Can you work these out from the model? Positions are in its coordinate system, mm. A direction names the side the tool comes from. Round coordinates to 2 decimals unless told otherwise and drop trailing zeros. Write each loop counter-clockwise with the first axis right and the second up, starting at its lowest first coordinate (ties: lowest second). Pieces come first, ordered by that corner, then holes. Notation, with made-up numbers: (32.5, 53.5) - (70.5, 53.5) arc R17 ccw to (70.5, 72.5) - close; hole circle Ø9 at (-22, 34). An arc over 180 degrees is marked (long way). One line per item, written item: value. Start each with the question number.
(1) If I drill on L1, parallel to Y at x = 0, z = 3.9; L2, parallel to Z at x = 2, y = -6; L3, parallel to Y at x = 0, z = 1.7, over which ranges is the centre line in solid material (lowest first)? Write a range as from..to.
(2) I want a section at D-D on z = 2.35. List the corners of the cut face in (x, y) for me, plus the area to 3 significant figures.
(3) I want a section at A-A on y = 0. List the corners of the cut face in (x, z) for me.
(4) On a 3-axis mill with a long thin cutter (end or side, diameter ignored), from which of +Z, -Z, +X, -X, +Y, -Y can I reach the whole of each face in a straight line? I mean faces 1 (the face through (4.3, -2.1, 0)), 2 (the face through (3.4, -3.4, 2.7)). Say none if no direction works.
(5) I want a section at C-C on z = 4.5. List the corners of the cut face in (x, y) for me, plus the area to 3 significant figures.
(6) I'm going to push flat-ended pins straight in: pin 1 Ø1 at (y, z) = (4.5, 4.5) entering from +X; pin 2 Ø11.5 at (x, y) = (0, 0) entering from +Z; pin 3 Ø3 at (y, z) = (4, 3) entering from +X; pin 4 Ø2 at (y, z) = (0.5, 2) entering from +X. Where does each tip first touch, or does it pass through?
(7) Thinking about a two-plate mould opening in Y: for faces 3 (the face through (-11.99, 0.53, 3.58)), 4 (the face through (-0.59, 4.46, 1.37)), 5 (the face through (-1.73, -7.81, 3.97)), 6 (the face through (2, -8, 5.2)), which applies, +Y half, -Y half, draft (parallel to the pull), parting line (faces both ways), or undercut?
from build123d import *

# Parameters (mm, degrees)
IZIM4_R                     = 12
Y_KSEKLIK_EKSTR_ZYON3_DEPTH = 5.2
IZIM6_R                     = 8
KES_EKSTR_ZYON2_DEPTH       = 2.5
IZIM7_R                     = 4.5
KES_EKSTR_ZYON3_DEPTH       = 12.6
PAH3_SIZE                   = 2


with BuildPart() as part:
    # Çizim4 → Yükseklik-Ekstrüzyon3 (new body)
    with BuildSketch(Plane.XY):
        Circle(IZIM4_R)
    extrude(amount=Y_KSEKLIK_EKSTR_ZYON3_DEPTH)

    # Çizim6 → Kes-Ekstrüzyon2 (cut)
    with BuildSketch(Plane.XY.offset(5.2)):
        Circle(IZIM6_R)
    extrude(amount=-KES_EKSTR_ZYON2_DEPTH, mode=Mode.SUBTRACT)

    # Çizim7 → Kes-Ekstrüzyon3 (cut)
    with BuildSketch(Plane.XY.offset(2.7)):
        Circle(IZIM7_R)
    extrude(amount=-KES_EKSTR_ZYON3_DEPTH, mode=Mode.SUBTRACT)

    # Pah3
    pah3_edges = [part.edges().sort_by_distance(p)[0] for p in [
        (-12, 0, 0),
    ]]
    chamfer(pah3_edges, length=PAH3_SIZE)


solid = part.part
Established:
1. L1: -12..-8, 8..12
1. L2: 0..2.7
1. L3: -11.7..-4.5, 4.5..11.7
2. outline: circle Ø24 at (0, 0); hole circle Ø9 at (0, 0)
2. area: 389 mm2
3. outline: (-12, 2) - (-10, 0) - (-4.5, 0) - (-4.5, 2.7) - (-8, 2.7) - (-8, 5.2) - (-12, 5.2) - close; (4.5, 0) - (10, 0) - (12, 2) - (12, 5.2) - (8, 5.2) - (8, 2.7) - (4.5, 2.7) - close
4. face 1: -Z, +X, -X, +Y, -Y
4. face 2: +Z
5. outline: circle Ø24 at (0, 0); hole circle Ø16 at (0, 0)
5. area: 251 mm2
6. pin 1: x = 11.31
6. pin 2: z = 2.7
6. pin 3: x = 11.74
6. pin 4: x = 12
7. face 3: parting line
7. face 4: undercut
7. face 5: undercut
7. face 6: draft
